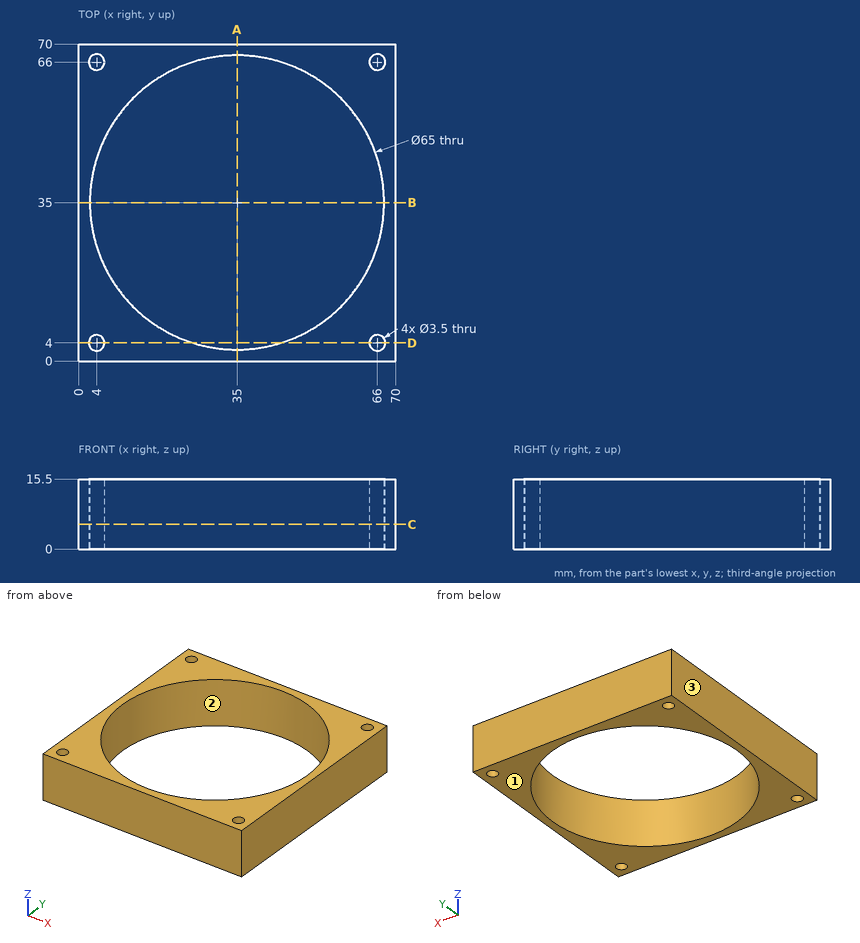
Answer from the drawing. Dimensions are ordinates in mm from the lowest x, y and z of the part. Coordinates: 2 decimals unless noted, no trailing zeros. Loops run counter-clockwise (first coordinate to the right, second up) from the corner with the lowest first, then second, coordinate; pieces in that order, holes last. Notation, with made-up numbers: (65.5, 52) - (102.5, 52) arc R33 cw to (102.5, 82) - close; hole circle Ø6 at (-34, -9). An arc over 180 degrees is marked (long way). Answer in a Markdown table with one row per item.
1. Given pin 1 (6 mm diameter, centred on x = 9.5, z = 4.5, fed in from -Y), flat-ended and moving along its own axis, determine where the tip first touches the part or whether it passes through.
Conclusion:
| item | result |
|---|---|
| pin 1 | stops at y = 0 |
2. Find section D-D, the plane y = 4. Write down the section's boundary in (x, z).
Conclusion:
| item | result |
|---|---|
| outline | (0, 0) - (2.25, 0) - (2.25, 15.5) - (0, 15.5) - close; (5.75, 0) - (25.24, 0) - (25.24, 15.5) - (5.75, 15.5) - close; (44.76, 0) - (64.25, 0) - (64.25, 15.5) - (44.76, 15.5) - close; (67.75, 0) - (70, 0) - (70, 15.5) - (67.75, 15.5) - close |
3. Straight lines are drawn through the part: line 1 (X direction, y = 65, z = 3.5); line 2 (Y direction, x = 30.5, z = 1.5); line 3 (Y direction, x = 35, z = 9.5). For each, find the intervals that lie inside material, in ascending order.
Conclusion:
| item | result |
|---|---|
| line 1 | x = 0 to 2.56, 5.44 to 22.5, 47.5 to 64.56, 67.44 to 70 |
| line 2 | y = 0 to 2.81, 67.19 to 70 |
| line 3 | y = 0 to 2.5, 67.5 to 70 |
4. Find section A-A, the plane x = 35. Write down the section's boundary in (y, z), then the cut area to 3 significant figures.
Conclusion:
| item | result |
|---|---|
| outline | (0, 0) - (2.5, 0) - (2.5, 15.5) - (0, 15.5) - close; (67.5, 0) - (70, 0) - (70, 15.5) - (67.5, 15.5) - close |
| area | 77.5 mm² |
5. Determine the mould class of the marked faces 1, 2 and 3 for opening direction X: +X half, -X half, draft (parallel to the pull), parting line (faces both ways), or undercut.
Conclusion:
| item | result |
|---|---|
| face 1 | draft |
| face 2 | undercut |
| face 3 | -X half |
6. Find section C-C, the plane z = 5.5. Write down the section's boundary in (x, y).
Conclusion:
| item | result |
|---|---|
| outline | (0, 0) - (70, 0) - (70, 70) - (0, 70) - close; hole circle Ø3.5 at (4, 4); hole circle Ø3.5 at (4, 66); hole circle Ø65 at (35, 35); hole circle Ø3.5 at (66, 4); hole circle Ø3.5 at (66, 66) |
